The model under review builds one solid part; all positions refer to its coordinate system, in mm. A direction names the side the tool comes from. Round coordinates to 2 decimals unless told otherwise and drop trailing zeros. Order: outer loops, then holes, each group sorted by start corner. A loop starts at its lowest first (then second) coordinate and runs counter-clockwise, first axis right, second up. Notation, with made-up numbers: M 33,81 L 81,81 A36 ccw 81,120 Z; hole C 33,75.25 d9. An arc over 180 degrees is marked long. Use a Markdown table: item, result. Add a question column.
1. Consider section C-C on y = 13. State the section outline as (x, z) points.
2. To check wall thickness, follow probe 1 along X at (y, z) = (1, 0); probe 2 along Z at (x, y) = (21, 10.5); probe 3 along X at (y, z) = (27, 19.5). State the ranges of each line that lie inside material, in increasing order.
3. Consider section D-D on z = 7. State the section outline as (x, y) points.
4. The part is to be moulded in two halves that separate along X. For faces 1 (the flat face through (-15, 2, 0)), 2 (the flat face through (0, 0, -5)), 3 (the flat face through (15, 2, 0)), say which applies: +X half, -X half, draft (parallel to the pull), parting line (faces both ways), or undercut.
5. Consider section A-A on x = 10. State the section outline as (y, z) points.
6. For faces 4 (the flat face through (0, -20, 36)), 5 (the flat face through (0, -15, 41)), 6 (the flat face through (-25, 25, 16)), 7 (the flat face through (30, 25.4, 16.4)), list the 3-axis set-ups (+Z, -Z, +X, -X, +Y, -Y) from which the entire face can be reached by the end or side of a thin tool; tool diameter is ignored.
7. Consider section B-B on z = 41. State the section outline as (x, y) points.
8. Insertion check: P1, Ø8, axis at x = -11.5, y = -8, coming from the +Z side; P2, Ø5.5, axis at x = -2.5, y = 3, coming from the +Z side; P3, Ø4, axis at y = 2.5, z = 0, coming from the +X side. Each pin has a flat end and moves straight along its axis. Give the tip position at first contact, or say it passes through.
from build123d import *

# Parameters (mm, degrees)
SKETCH_1_W           = 30
SKETCH_1_H           = 18
SKETCH_1_R           = 1.35
EXTRUDE_1_DEPTH      = 5
SKETCH_2_W           = 60
SKETCH_2_H           = 60
SKETCH_2_W_2         = 40
SKETCH_2_H_2         = 40
EXTRUDE_2_DEPTH      = 30
EXTRUDE_2_DEPTH_BACK = 30
SKETCH_3_W           = 40
SKETCH_3_H           = 40
CUT_EXTRUDE_1_DEPTH  = 10
SKETCH_4_W           = 40
SKETCH_4_H           = 40
CUT_EXTRUDE_2_DEPTH  = 10
SKETCH_5_W           = 40
SKETCH_5_H           = 40
CUT_EXTRUDE_3_DEPTH  = 10
SKETCH_6_W           = 40
SKETCH_6_H           = 20
SKETCH_6_H_2         = 15
CUT_EXTRUDE_4_DEPTH  = 10
CHAMFER_1_SIZE       = 5


with BuildPart() as part:
    # 스케치1 → 보스-돌출1 (new body)
    with BuildSketch(Plane(origin=(0, 0, 0), x_dir=(1, 0, 0), z_dir=(0, 1, 0))):
        with Locations((0, 5)):
            Rectangle(SKETCH_1_W, SKETCH_1_H)
        with Locations((-10, 0)):
            Circle(SKETCH_1_R, mode=Mode.SUBTRACT)
        with Locations((10, 0)):
            Circle(SKETCH_1_R, mode=Mode.SUBTRACT)
    extrude(amount=EXTRUDE_1_DEPTH)

    # 스케치2 → 보스-돌출2 (add, two sides)
    with BuildSketch(Plane(origin=(0, 5, 0), x_dir=(1, 0, 0), z_dir=(0, 1, 0))) as extrude_2_sk:
        with Locations((0, -16)):
            Rectangle(SKETCH_2_W, SKETCH_2_H)
        with Locations((0, -16)):
            Rectangle(SKETCH_2_W_2, SKETCH_2_H_2, mode=Mode.SUBTRACT)
    extrude(amount=EXTRUDE_2_DEPTH)
    extrude(extrude_2_sk.sketch, amount=-EXTRUDE_2_DEPTH_BACK)

    # 스케치3 → 컷-돌출1 (cut)
    with BuildSketch(Plane.XY.offset(46)):
        with Locations((0, 5)):
            Rectangle(SKETCH_3_W, SKETCH_3_H)
    extrude(amount=-CUT_EXTRUDE_1_DEPTH, mode=Mode.SUBTRACT)

    # 스케치4 → 컷-돌출2 (cut)
    with BuildSketch(Plane.ZY.offset(30)):
        with Locations((16, 5)):
            Rectangle(SKETCH_4_W, SKETCH_4_H)
    extrude(amount=-CUT_EXTRUDE_2_DEPTH, mode=Mode.SUBTRACT)

    # 스케치5 → 컷-돌출3 (cut)
    with BuildSketch(Plane(origin=(30, 0, 0), x_dir=(0, 0, -1), z_dir=(1, 0, 0))):
        with Locations((-16, 5)):
            Rectangle(SKETCH_5_W, SKETCH_5_H)
    extrude(amount=-CUT_EXTRUDE_3_DEPTH, mode=Mode.SUBTRACT)

    # 스케치6 → 컷-돌출4 (cut)
    with BuildSketch(Plane.XY.offset(-4)):
        with Locations((0, 15)):
            Rectangle(SKETCH_6_W, SKETCH_6_H)
        with Locations((0, -7.5)):
            Rectangle(SKETCH_6_W, SKETCH_6_H_2)
    extrude(amount=-CUT_EXTRUDE_4_DEPTH, mode=Mode.SUBTRACT)

    # 모따기1
    chamfer_1_edges = [part.edges().sort_by_distance(p)[0] for p in [
        (20, 5, -9),
        (-20, 5, -9),
        (-20, 0, -9),
        (20, 0, -9),
    ]]
    chamfer(chamfer_1_edges, length=CHAMFER_1_SIZE)


solid = part.part
Answer block:
| question | item | result |
|---|---|---|
| 1 | outline | M -30,-14 L -20,-14 L -20,-4 L -30,-4 Z; M -30,36 L -20,36 L -20,46 L -30,46 Z; M 20,-14 L 30,-14 L 30,-4 L 20,-4 Z; M 20,36 L 30,36 L 30,46 L 20,46 Z |
| 2 | probe 1 | -15 to -11.35, -8.65 to 8.65, 11.35 to 15 |
| 2 | probe 2 | -14 to -4, 36 to 46 |
| 2 | probe 3 | -30 to -20, 20 to 30 |
| 3 | outline | M -30,-25 L -20,-25 L -20,-15 L -30,-15 Z; M -30,25 L -20,25 L -20,35 L -30,35 Z; M 20,-25 L 30,-25 L 30,-15 L 20,-15 Z; M 20,25 L 30,25 L 30,35 L 20,35 Z |
| 4 | face 1 | -X half |
| 4 | face 2 | undercut |
| 4 | face 3 | +X half |
| 5 | outline | M -25,-14 L -15,-14 L -15,-4 L -25,-4 Z; M -25,36 L -15,36 L -15,46 L -25,46 Z; M 0,-14 L 5,-14 L 5,-1.35 L 0,-1.35 Z; M 0,1.35 L 5,1.35 L 5,4 L 0,4 Z; M 25,-14 L 35,-14 L 35,-4 L 25,-4 Z; M 25,36 L 35,36 L 35,46 L 25,46 Z |
| 6 | face 4 | +Y, -Y |
| 6 | face 5 | +Z, -Z |
| 6 | face 6 | +X, -X |
| 6 | face 7 | +Z, -Z, +X, +Y, -Y |
| 7 | outline | M -30,-25 L 30,-25 L 30,35 L -30,35 Z; hole M -20,-15 L 20,-15 L 20,25 L -20,25 Z |
| 8 | P1 | through |
| 8 | P2 | z = 4 |
| 8 | P3 | x = 15 |
